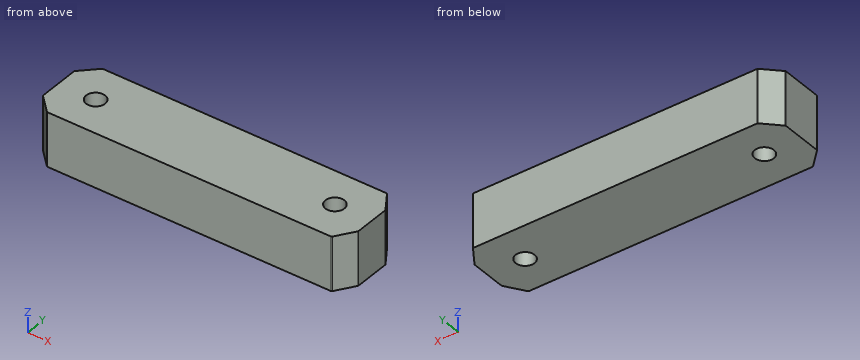
from build123d import *

# Parameters (mm, degrees)
SKETCH1_R           = 1.666
BOSS_EXTRUDE1_DEPTH = 9.45


with BuildPart() as part:
    # Sketch1 → Boss-Extrude1 (new body)
    with BuildSketch(Plane.XY):
        with BuildLine():
            Line((-24.730151519, -6.441421356), (-27.441421356, -3.730151519))
            ThreePointArc((-27.441421356, -3.730151519), (-27.484775907, -3.665266849), (-27.5, -3.588730163))
            Line((-27.5, -3.588730163), (-27.5, 3.588730163))
            ThreePointArc((-27.5, 3.588730163), (-27.484775907, 3.665266849), (-27.441421356, 3.730151519))
            Line((-27.441421356, 3.730151519), (-24.730151519, 6.441421356))
            ThreePointArc((-24.730151519, 6.441421356), (-24.665266849, 6.484775907), (-24.588730163, 6.5))
            Line((-24.588730163, 6.5), (25.17448832, 6.5))
            ThreePointArc((25.17448832, 6.5), (25.268868885, 6.476330114), (25.340909677, 6.410923091))
            Line((25.340909677, 6.410923091), (27.466421356, 3.221951957))
            Line((27.466421356, 3.221951957), (27.5, 3.111028865))
            Line((27.5, 3.111028865), (27.5, -3.111028865))
            Line((27.5, -3.111028865), (27.466421356, -3.221951957))
            Line((27.466421356, -3.221951957), (25.340909677, -6.410923091))
            ThreePointArc((25.340909677, -6.410923091), (25.268868885, -6.476330114), (25.17448832, -6.5))
            Line((25.17448832, -6.5), (-24.588730163, -6.5))
            ThreePointArc((-24.588730163, -6.5), (-24.665266849, -6.484775907), (-24.730151519, -6.441421356))
        make_face()
        with Locations((21, 0)):
            Circle(SKETCH1_R, mode=Mode.SUBTRACT)
        with Locations((-21, 0)):
            Circle(SKETCH1_R, mode=Mode.SUBTRACT)
    extrude(amount=BOSS_EXTRUDE1_DEPTH)


solid = part.part
Could you check a few things on this model? Use its own coordinates, in mm. Coordinates: 2 decimals unless noted, no trailing zeros. Write each loop counter-clockwise with the first axis right and the second up, starting at its lowest first coordinate (ties: lowest second). Pieces come first, ordered by that corner, then holes. Notation, with made-up numbers: M 29.5,44.25 L 85.5,44.25 A26 ccw 85.5,59.25 Z; hole C -21,81 d2. An arc over 180 degrees is marked long. One line per question, with ' | ' between items.
1) Imagine slicing it at C-C, the plane z = 5.25. Write out the boundary of the cut face in (x, y).
Checks:
outline: M -27.5,-3.59 A0.2 ccw -27.44,-3.73 L -24.73,-6.44 A0.2 ccw -24.59,-6.5 L 25.17,-6.5 A0.2 ccw 25.34,-6.41 L 27.47,-3.22 L 27.5,-3.11 L 27.5,3.11 L 27.47,3.22 L 25.34,6.41 A0.2 ccw 25.17,6.5 L -24.59,6.5 A0.2 ccw -24.73,6.44 L -27.44,3.73 A0.2 ccw -27.5,3.59 Z; hole C -21,0 d3.33; hole C 21,0 d3.33
2) For pin 1 Ø4 at (x, y) = (21, 0) entering from +Z; pin 2 Ø2.5 at (x, y) = (-21, 0) entering from +Z; pin 3 Ø1 at (y, z) = (-4, 5) entering from +X, each with a flat end and sliding along its axis, tell me the tip position at first contact or that it passes through.
Checks:
pin 1: z = 9.45 | pin 2: through | pin 3: x = 27.28
3) Imagine slicing it at A-A, the plane x = -21. Write out the boundary of the cut face in (y, z).
Checks:
outline: M -6.5,0 L -1.67,0 L -1.67,9.45 L -6.5,9.45 Z; M 1.67,0 L 6.5,0 L 6.5,9.45 L 1.67,9.45 Z
4) I need wall thicknesses on probe 1 along Y at (x, z) = (-21, 5.5); probe 2 along X at (y, z) = (1, 3); probe 3 along X at (y, z) = (1.5, 2.5). Which ranges of each line are inside material? Lowest first, please. Write a range as [from, to].
Checks:
probe 1: [-6.5, -1.67], [1.67, 6.5] | probe 2: [-27.5, -22.33], [-19.67, 19.67], [22.33, 27.5] | probe 3: [-27.5, -21.72], [-20.28, 20.28], [21.72, 27.5]
5) Imagine slicing it at B-B, the plane y = 0. Write out the boundary of the cut face in (x, z).
Checks:
outline: M -27.5,0 L -22.67,0 L -22.67,9.45 L -27.5,9.45 Z; M -19.33,0 L 19.33,0 L 19.33,9.45 L -19.33,9.45 Z; M 22.67,0 L 27.5,0 L 27.5,9.45 L 22.67,9.45 Z
6) Imagine slicing it at D-D, the plane y = 5. Write out the boundary of the cut face in (x, z).
Checks:
outline: M -26.17,0 L 26.28,0 L 26.28,9.45 L -26.17,9.45 Z
